Drawing for the job (mm, zero at the part's lowest x, y, z). Coordinates: 2 decimals unless noted, no trailing zeros. Order: outer loops, then holes, each group sorted by start corner. A loop starts at its lowest first (then second) coordinate and runs counter-clockwise, first axis right, second up. Notation, with made-up numbers: (30, 50.5) -> (66, 50.5) arc R20 ccw to (66, 75.5) -> close; hole circle Ø9 at (-24.5, 22.25). An arc over 180 degrees is marked (long way). Write each question's results on one line, items separated by ' | '.
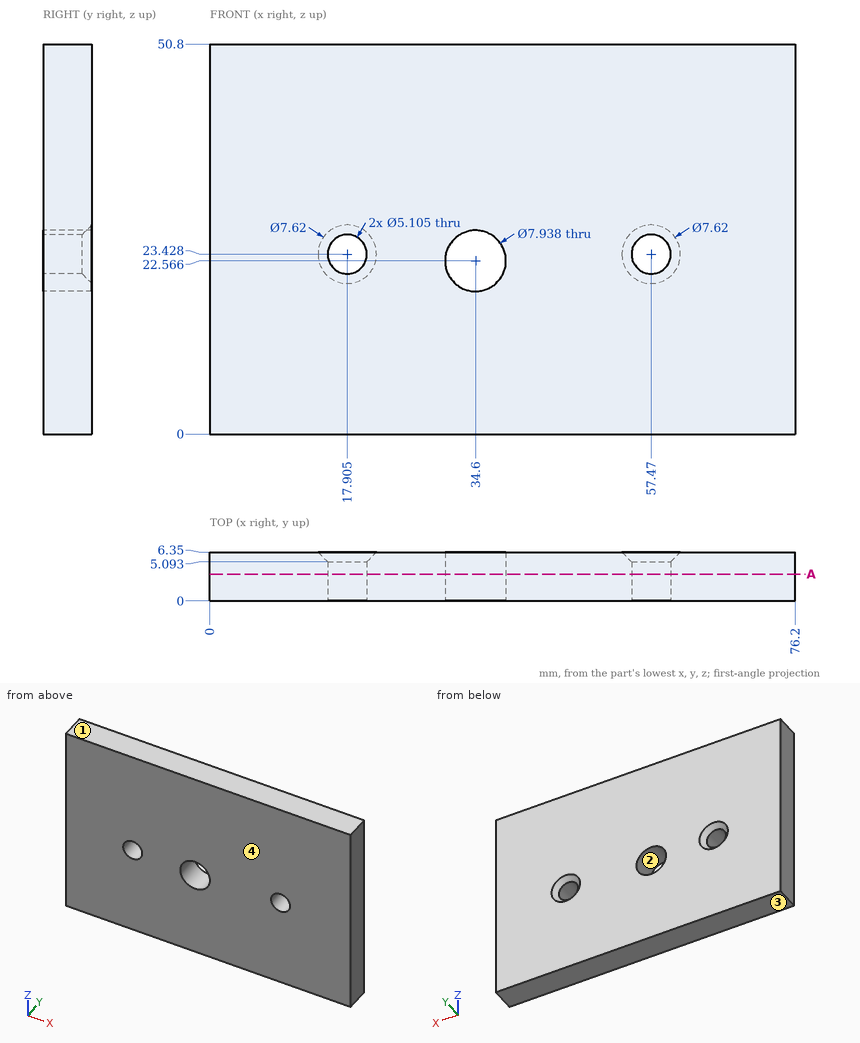
Item 1: Pin check, flat tips, straight feed: pin 1 (6.5 mm diameter, centred on x = 17.91, z = 23.43, fed in from +Y) (1 decimal); pin 2 (3 mm diameter, centred on y = 1.5, z = 35.5, fed in from -X); pin 3 (6 mm diameter, centred on x = 57.47, z = 23.43, fed in from +Y); pin 4 (5 mm diameter, centred on x = 34.6, z = 22.57, fed in from +Y). Stop position of each tip, or through.
Answer:
pin 1: stops at y = 5.8 | pin 2: stops at x = 0 | pin 3: stops at y = 5.54 | pin 4: passes through
Item 2: Drill centre lines: line 1 (X direction, y = 3.75, z = 23.5) (1 decimal); line 2 (Z direction, x = 58.5, y = 1.5) (1 decimal); line 3 (X direction, y = 3.5, z = 24.5) (1 decimal). Where is each one in solid material? Low to high. Write a range as from..to.
Answer:
line 1: x = 0..15.4, 20.5..30.7, 38.5..54.9, 60..76.2 | line 2: z = 0..21.1, 25.8..50.8 | line 3: x = 0..15.6, 20.2..31.1, 38.1..55.2, 59.8..76.2
Item 3: Slice it at A-A, the plane y = 3.5. List the corners of the cut face in (x, z) (1 decimal), and give its area (3 significant figures).
Answer:
outline: (0, 0) -> (76.2, 0) -> (76.2, 50.8) -> (0, 50.8) -> close; hole circle Ø5.1 at (17.9, 23.4); hole circle Ø7.9 at (34.6, 22.6); hole circle Ø5.1 at (57.5, 23.4) | area: 3,780 mm^2
Item 4: Pull direction Z, two halves, no side cores. Call the marked faces 1, 2, 3 and 4: released by +Z, released by -Z, zero draft, split by the parting line, or undercut.
Answer:
face 1: released by +Z | face 2: undercut | face 3: released by -Z | face 4: zero draft
